Verification items for the finished model (mm, model axes). A direction names the side the tool comes from. Coordinates: 2 decimals unless noted, no trailing zeros. Loops run counter-clockwise (first coordinate to the right, second up) from the corner with the lowest first, then second, coordinate; pieces in that order, holes last. Notation, with made-up numbers: (-1.75, -13.5) - (54.25, -13.5) arc R21 ccw to (54.25, -0.5) - close; hole circle Ø5 at (85.25, 18.5). An arc over 180 degrees is marked (long way). Answer as CSV lines item,"result". Start each with the question number.
1. Cross-section at B-B (x = 27.5). Enter the section's corners in (y, z).
2. Gauge pin test, flat ends, axial feed: P1, Ø12, axis at y = 15, z = 49, coming from the -X side; P2, Ø4, axis at x = 51, z = -1.71, coming from the +Y side; P3, Ø5, axis at x = 26.5, y = 18.5, coming from the +Z side; P4, Ø6.5, axis at x = 0.5, z = -3, coming from the +Y side. Record the tip position at first contact, or that the pin passes through.
3. Material ranges on line 1 (Z direction, x = -1, y = -24.6); line 2 (X direction, y = 6, z = 7.5); line 3 (Z direction, x = 6, y = -2), recorded low to high. Write a range as [from, to].
4. Set-up check for faces 4 (the flat face through (47, -1, 1)), 5 (the flat face through (-1, -23, 2)), 6 (the flat face through (43, -15, 10)), 7 (the cylindrical face through (-3.385, -23.986, -0.96)): record each of +Z, -Z, +X, -X, +Y, -Y from which the full face is reachable in a straight line by a thin tool's end or side.
5. Cross-section at D-D (y = -12). Enter the section's corners in (x, z).
6. Cross-section at A-A (z = 30). Enter the section's corners in (x, y), plus the area to 3 significant figures.
7. Cross-section at C-C (x = 15.5). Enter the section's corners in (y, z).
8. Release check for a two-part mould opening along Z. For faces 1 (the cylindrical face through (48.69, -23.99, -2.67)), 2 (the cylindrical face through (4.31, -0.93, 6.77)), 3 (the flat face through (21.25, 20, 30)) record: pulls with the +Z half, pulls with the -Z half, needs draft (parallel to the pull), parting line crosses it, or undercut.
```python
from build123d import *

# Parameters (mm, degrees)
BOSS_EXTRUDE1_DEPTH = 50
SKETCH3_R           = 4.25
CUT_EXTRUDE2_DEPTH  = 90.866567755
SKETCH5_W           = 10
SKETCH5_H           = 5
BOSS_EXTRUDE2_DEPTH = 16
FILLET1_R           = 2
SKETCH6_W           = 2.5
SKETCH6_H           = 7.68
CUT_EXTRUDE3_DEPTH  = 16
SKETCH9_W           = 50
SKETCH9_H           = 22.289567514
CUT_EXTRUDE4_DEPTH  = 92.520489509
SKETCH10_W          = 60
SKETCH10_H          = 54
BOSS_EXTRUDE3_DEPTH = 5
SKETCH11_W          = 23
SKETCH11_H          = 24
SKETCH11_W_2        = 36
CUT_EXTRUDE5_DEPTH  = 5
SKETCH12_W          = 8
SKETCH12_H          = 4
BOSS_EXTRUDE4_DEPTH = 13
FILLET2_R           = 3
FILLET3_R           = 3
FILLET4_R           = 3
FILLET5_R           = 3
SKETCH13_R          = 2.5
CUT_EXTRUDE6_DEPTH  = 13
SKETCH14_R          = 2.5
CUT_EXTRUDE7_DEPTH  = 10
SKETCH15_R          = 2.5
CUT_EXTRUDE8_DEPTH  = 2


with BuildPart() as part:
    # Sketch2 → Boss-Extrude1 (new body)
    with BuildSketch(Plane(origin=(0, 0, 0), x_dir=(0, 0, -1), z_dir=(1, 0, 0))):
        with BuildLine():
            Line((-74, 10), (0, 10))
            ThreePointArc((0, 10), (10, 0), (0, -10))
            Line((0, -10), (-74, -10))
            Line((-74, -10), (-74, 10))
        make_face()
    extrude(amount=BOSS_EXTRUDE1_DEPTH)

    # Sketch3 → Cut-Extrude2 (cut, through all)
    with BuildSketch(Plane(origin=(50, 0, 0), x_dir=(0, 0, -1), z_dir=(1, 0, 0))):
        with Locations((-30, 0)):
            Circle(SKETCH3_R)
        with Locations((-50, 0)):
            Circle(SKETCH3_R)
    extrude(amount=-CUT_EXTRUDE2_DEPTH, mode=Mode.SUBTRACT)

    # Sketch5 → Boss-Extrude2 (add)
    with BuildSketch(Plane(origin=(0, 10, 0), x_dir=(1, 0, 0), z_dir=(0, 1, 0))):
        with Locations((25, -30)):
            Rectangle(SKETCH5_W, SKETCH5_H)
    extrude(amount=BOSS_EXTRUDE2_DEPTH)

    # Fillet1
    fillet1_edges = [part.edges().sort_by_distance(p)[0] for p in [
        (25, 10, 27.5),
    ]]
    fillet(fillet1_edges, radius=FILLET1_R)

    # Sketch6 → Cut-Extrude3 (cut)
    with BuildSketch(Plane.XY.offset(32.5)):
        with Locations((22.5, 20.5)):
            Rectangle(SKETCH6_W, SKETCH6_H)
        with Locations((27.5, 20.5)):
            Rectangle(SKETCH6_W, SKETCH6_H)
    extrude(amount=-CUT_EXTRUDE3_DEPTH, mode=Mode.SUBTRACT)

    # Sketch9 → Cut-Extrude4 (cut, through all)
    with BuildSketch(Plane(origin=(0, 10, 0), x_dir=(1, 0, 0), z_dir=(0, 1, 0))):
        with Locations((25, -1.144783757)):
            Rectangle(SKETCH9_W, SKETCH9_H)
    extrude(amount=-CUT_EXTRUDE4_DEPTH, mode=Mode.SUBTRACT)

    # Sketch10 → Boss-Extrude3 (add)
    with BuildSketch(Plane(origin=(0, 0, 12.289567514), x_dir=(-1, 0, 0), z_dir=(0, 0, -1))):
        with Locations((-25, 0)):
            Rectangle(SKETCH10_W, SKETCH10_H)
    extrude(amount=BOSS_EXTRUDE3_DEPTH)

    # Sketch11 → Cut-Extrude5 (cut)
    with BuildSketch(Plane(origin=(0, 0, 7.289567514), x_dir=(-1, 0, 0), z_dir=(0, 0, -1))):
        with Locations((-25, 12)):
            Rectangle(SKETCH11_W, SKETCH11_H)
        with Locations((-25, -15)):
            Rectangle(SKETCH11_W_2, SKETCH11_H)
    extrude(amount=-CUT_EXTRUDE5_DEPTH, mode=Mode.SUBTRACT)

    # Sketch12 → Boss-Extrude4 (add)
    with BuildSketch(Plane(origin=(0, 0, 7.289567514), x_dir=(-1, 0, 0), z_dir=(0, 0, -1))):
        with Locations((1, 25)):
            Rectangle(SKETCH12_W, SKETCH12_H)
        with Locations((-51, 25)):
            Rectangle(SKETCH12_W, SKETCH12_H)
        with Locations((1, -25)):
            Rectangle(SKETCH12_W, SKETCH12_H)
        with Locations((-51, -25)):
            Rectangle(SKETCH12_W, SKETCH12_H)
        with Locations((1, -1)):
            Rectangle(SKETCH12_W, SKETCH12_H)
        with Locations((-51, -1)):
            Rectangle(SKETCH12_W, SKETCH12_H)
    extrude(amount=BOSS_EXTRUDE4_DEPTH)

    # Fillet2
    fillet2_edges = [part.edges().sort_by_distance(p)[0] for p in [
        (-5, 25, -5.710432486),
        (3, 25, -5.710432486),
        (55, 25, -5.710432486),
        (47, 25, -5.710432486),
        (-5, -25, -5.710432486),
        (3, -25, -5.710432486),
        (55, -25, -5.710432486),
        (47, -25, -5.710432486),
        (-5, -1, -5.710432486),
        (3, -1, -5.710432486),
        (55, -1, -5.710432486),
        (47, -1, -5.710432486),
    ]]
    fillet(fillet2_edges, radius=FILLET2_R)

    # Fillet3
    fillet3_edges = [part.edges().sort_by_distance(p)[0] for p in [
        (3, 25, 7.289567514),
        (-1, 23, 7.289567514),
    ]]
    fillet(fillet3_edges, radius=FILLET3_R)

    # Fillet4
    fillet4_edges = [part.edges().sort_by_distance(p)[0] for p in [
        (51, 23, 7.289567514),
        (47, 25, 7.289567514),
        (-1, -23, 7.289567514),
        (3, -25, 7.289567514),
        (47, -25, 7.289567514),
        (51, -23, 7.289567514),
        (3, -1, 7.289567514),
        (-1, -3, 7.289567514),
        (51, -3, 7.289567514),
        (47, -1, 7.289567514),
    ]]
    fillet(fillet4_edges, radius=FILLET4_R)

    # Fillet5
    fillet5_edges = [part.edges().sort_by_distance(p)[0] for p in [
        (49.5, 1, 7.289567514),
        (0.5, 1, 7.289567514),
    ]]
    fillet(fillet5_edges, radius=FILLET5_R)

    # Sketch13 → Cut-Extrude6 (cut)
    with BuildSketch(Plane(origin=(0, 27, 0), x_dir=(1, 0, 0), z_dir=(0, 1, 0))):
        with Locations(Location((51, 1.710432486, 0), (0, 0, 180))):
            Circle(SKETCH13_R)
        with Locations(Location((-1, 1.710432486, 0), (0, 0, 180))):
            Circle(SKETCH13_R)
    extrude(amount=-CUT_EXTRUDE6_DEPTH, mode=Mode.SUBTRACT)

    # Sketch14 → Cut-Extrude7 (cut)
    with BuildSketch(Plane(origin=(0, 1, 0), x_dir=(1, 0, 0), z_dir=(0, 1, 0))):
        with Locations(Location((51, 1.710432486, 0), (0, 0, 180))):
            Circle(SKETCH14_R)
        with Locations(Location((-1, 1.710432486, 0), (0, 0, 180))):
            Circle(SKETCH14_R)
    extrude(amount=-CUT_EXTRUDE7_DEPTH, mode=Mode.SUBTRACT)

    # Sketch15 → Cut-Extrude8 (cut)
    with BuildSketch(Plane(origin=(0, -23, 0), x_dir=(1, 0, 0), z_dir=(0, 1, 0))):
        with Locations(Location((51, 1.710432486, 0), (0, 0, 180))):
            Circle(SKETCH15_R)
        with Locations(Location((-1, 1.710432486, 0), (0, 0, 180))):
            Circle(SKETCH15_R)
    extrude(amount=-CUT_EXTRUDE8_DEPTH, mode=Mode.SUBTRACT)


solid = part.part
```
Values follow:
1,outline,"(-10, 12.29) - (-3, 12.29) - (-3, 7.29) - (0, 7.29) - (0, 12.29) - (10, 12.29) - (10, 25.5) arc R2 cw to (12, 27.5) - (16.66, 27.5) - (16.66, 32.5) - (10, 32.5) - (10, 74) - (-10, 74) - close; (24, 7.29) - (27, 7.29) - (27, 12.29) - (24, 12.29) - close; (24.34, 27.5) - (26, 27.5) - (26, 32.5) - (24.34, 32.5) - close; hole circle Ø8.5 at (0, 30); hole circle Ø8.5 at (0, 50)"
2,P1,"stops at x = 0"
2,P2,"stops at y = -25"
2,P3,"stops at z = 32.5"
2,P4,"stops at y = 27"
3,line 1,"z = [-5.71, -4.21], [0.79, 12.29]"
3,line 2,"x = [-5, 13.5], [36.5, 55]"
3,line 3,"z = [7.29, 26.25], [33.75, 46.25], [53.75, 74]"
4,face 4,"-Z, +Y, -Y"
4,face 5,"-Z, +X, -X"
4,face 6,"-Z, -Y"
4,face 7,"+Y"
5,outline,"(-5, 7.29) - (7, 7.29) - (7, 12.29) - (-5, 12.29) - close; (43, 7.29) - (55, 7.29) - (55, 12.29) - (43, 12.29) - close"
6,outline,"(0, -10) - (50, -10) - (50, -4.25) - (0, -4.25) - close; (0, 4.25) - (50, 4.25) - (50, 10) - (30, 10) - (30, 26) - (20, 26) - (20, 10) - (0, 10) - close; hole (21.25, 16.66) - (23.75, 16.66) - (23.75, 24.34) - (21.25, 24.34) - close; hole (26.25, 16.66) - (28.75, 16.66) - (28.75, 24.34) - (26.25, 24.34) - close"
6,area,"697 mm²"
7,outline,"(-10, 12.29) - (-3, 12.29) - (-3, 7.29) - (0, 7.29) - (0, 12.29) - (10, 12.29) - (10, 74) - (-10, 74) - close; (24, 7.29) - (27, 7.29) - (27, 12.29) - (24, 12.29) - close; hole circle Ø8.5 at (0, 30); hole circle Ø8.5 at (0, 50)"
8,face 1,"undercut"
8,face 2,"pulls with the -Z half"
8,face 3,"needs draft"
